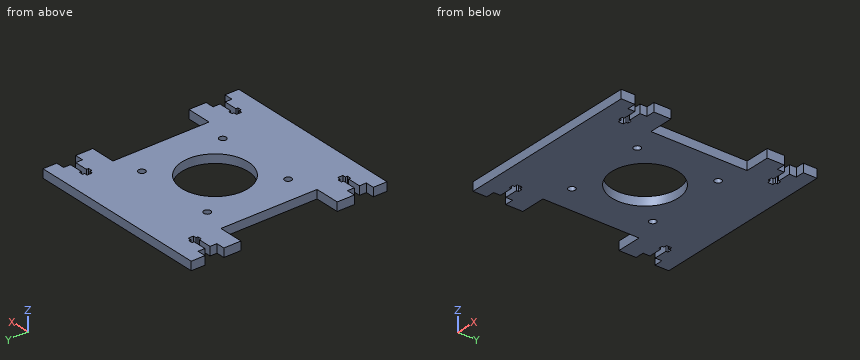
from build123d import *

# Parameters (mm, degrees)
MODEL_R                  = 2
MODEL_R_2                = 19.25
RESSALTO_EXTRUS_O1_DEPTH = 5


with BuildPart() as part:
    # Model → Ressalto-extrusão1 (new body)
    with BuildSketch(Plane.XY):
        Polygon((-87.499906276, 136.999930927), (-79.699992019, 136.999930927), (-79.699992019, 135.799931225), (-77.299992019, 135.799931225), (-77.299992019, 136.999930927), (-75.499992019, 136.999930927), (-75.499992019, 139.999946471), (-77.299992019, 139.999946471), (-77.299992019, 141.199946173), (-79.699992019, 141.199946173), (-79.699992019, 139.999946471), (-87.499906276, 139.999946471), (-87.499906276, 143.971527937), (-92.499906103, 143.971527937), (-92.499906103, 151.99992515), (14.500094446, 151.99992515), (14.500094446, 143.999926549), (9.500094619, 143.999926549), (9.500094619, 139.999946471), (1.700033295, 139.999946471), (1.700033295, 141.199946173), (-0.699966705, 141.199946173), (-0.699966705, 139.999946471), (-2.499966705, 139.999946471), (-2.499966705, 136.999930927), (-0.699966705, 136.999930927), (-0.699966705, 135.799931225), (1.700033295, 135.799931225), (1.700033295, 136.999930927), (9.500094619, 136.999930927), (9.500094619, 133.000010759), (14.500094446, 133.000010759), (14.500094446, 123.000010744), (3.1755e-05, 123.000010744), (3.1755e-05, 66.999892416), (14.500094446, 66.999892416), (14.500094446, 56.999892401), (9.500094619, 56.999892401), (9.500094619, 52.999972233), (1.700033295, 52.999972233), (1.700033295, 54.199971935), (-0.699966705, 54.199971935), (-0.699966705, 52.999972233), (-2.499966705, 52.999972233), (-2.499966705, 50.000008094), (-0.699966705, 50.000008094), (-0.699966705, 48.799928912), (1.700033295, 48.799928912), (1.700033295, 50.000008094), (9.500094619, 50.000008094), (9.500094619, 46.000008447), (14.500094446, 46.000008447), (14.500094446, 38.000009846), (-92.499906103, 38.000009846), (-92.499906103, 46.000008447), (-87.499906276, 46.000008447), (-87.499906276, 49.999928614), (-79.699992019, 49.999928614), (-79.699992019, 48.799928912), (-77.299992019, 48.799928912), (-77.299992019, 49.999928614), (-75.499992019, 49.999928614), (-75.499992019, 52.999972233), (-77.299992019, 52.999972233), (-77.299992019, 54.199971935), (-79.699992019, 54.199971935), (-79.699992019, 52.999972233), (-87.499906276, 52.999972233), (-87.499906276, 56.999892401), (-92.500404317, 56.999892401), (-92.500404317, 66.999892416), (-78.000001989, 66.999892416), (-78.000001989, 123.000010744), (-92.499906103, 123.000010744), (-92.499906103, 133.000010759), (-87.499906276, 133.000010759), align=None)
        with Locations((-62.569893888, 118.570002461)):
            Circle(MODEL_R, mode=Mode.SUBTRACT)
        with Locations((-15.429893888, 118.570002461)):
            Circle(MODEL_R, mode=Mode.SUBTRACT)
        with Locations((-62.569893888, 71.430002461)):
            Circle(MODEL_R, mode=Mode.SUBTRACT)
        with Locations((-15.429893888, 71.430002461)):
            Circle(MODEL_R, mode=Mode.SUBTRACT)
        with Locations((-38.999893888, 95.000002461)):
            Circle(MODEL_R_2, mode=Mode.SUBTRACT)
    extrude(amount=RESSALTO_EXTRUS_O1_DEPTH)


solid = part.part
Work out the finished part from the listing and answer in its coordinate system (mm). Round coordinates to 2 decimals unless told otherwise and drop trailing zeros. Write each loop counter-clockwise with the first axis right and the second up, starting at its lowest first coordinate (ties: lowest second). Pieces come first, ordered by that corner, then holes. Notation, with made-up numbers: (-40, 65) -> (-9, 65) arc R25 cw to (-9, 77) -> close; hole circle Ø3 at (74, 65.25). An arc over 180 degrees is marked (long way). Write each question's results on one line, items separated by ' | '.
Item 1: A flat-ended cylindrical pin translates along its axis: P1, Ø0.6, axis at y = 54, z = 1.5, coming from the +X side. Find the tip coordinate at first contact, or state that the pin passes through.
Result set:
P1: x = 9.5
Item 2: A cutting plane is placed at C-C, the plane x = -56.5. Determine the outline of the cut face in (y, z), plus the area to 3 significant figures.
Result set:
outline: (38, 0) -> (86.98, 0) -> (86.98, 5) -> (38, 5) -> close; (103.02, 0) -> (152, 0) -> (152, 5) -> (103.02, 5) -> close | area: 490 mm^2
Item 3: A cutting plane is placed at A-A, the plane x = -81. Determine the outline of the cut face in (y, z).
Result set:
outline: (38, 0) -> (50, 0) -> (50, 5) -> (38, 5) -> close; (53, 0) -> (67, 0) -> (67, 5) -> (53, 5) -> close; (123, 0) -> (137, 0) -> (137, 5) -> (123, 5) -> close; (140, 0) -> (152, 0) -> (152, 5) -> (140, 5) -> close
Item 4: A cutting plane is placed at B-B, the plane y = 85.5. Determine the outline of the cut face in (x, z).
Result set:
outline: (-78, 0) -> (-55.74, 0) -> (-55.74, 5) -> (-78, 5) -> close; (-22.26, 0) -> (0, 0) -> (0, 5) -> (-22.26, 5) -> close
Item 5: A cutting plane is placed at D-D, the plane z = 2.2. Count the separate pieces of the cut face and the enclosed holes in it, plus the area to 3 significant figures.
Result set:
separate pieces: 1 | enclosed holes: 5 | area: 8,970 mm^2
Item 6: Find the intervals of material crossed by line 1 along Y through (x, z) = (10, 0.7); line 2 along Y through (x, z) = (-15, 4.6); line 3 along Y through (x, z) = (-14, 1.55), in increasing order. Write a range as [from, to].
Result set:
line 1: [38, 46], [57, 67], [123, 133], [144, 152] | line 2: [38, 69.48], [73.38, 116.62], [120.52, 152] | line 3: [38, 70.03], [72.83, 117.17], [119.97, 152]
